CAD build for the part. Positions are in the model's coordinates, mm. Face numbers are marked on the shaded views. A direction names the side the tool comes from. Coordinates: 2 decimals unless noted, no trailing zeros. Write each loop counter-clockwise with the first axis right and the second up, starting at its lowest first coordinate (ties: lowest second). Pieces come first, ordered by that corner, then holes. Notation, with made-up numbers: (86.25, -30.75) -> (140.25, -30.75) arc R9 cw to (140.25, -15.75) -> close; hole circle Ø10 at (25.25, -24). An arc over 180 degrees is marked (long way). Answer as CSV lines item,"result".
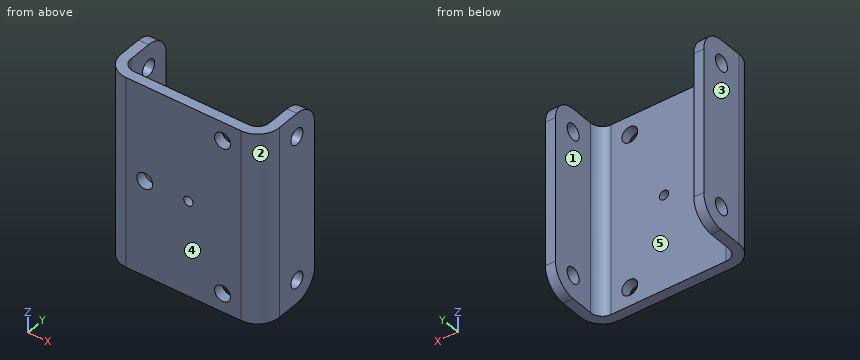
```python
from build123d import *

# Parameters (mm, degrees)
F1_DEPTH = 32.5777606
F2_R     = 3.69316
F3_R     = 1.98374
F4_R     = 1.35255
F5_DEPTH = 26.9875
F6_R     = 3.96875
F7_R     = 0.79375
F7_R_2   = 1.35255
F8_DEPTH = 1.70942


with BuildPart() as f1:
    # F0 (on Top) → F1 (new body)
    with BuildSketch(Plane.XY):
        Polygon((0, 9.92124), (0, 0), (-23.56866, 0), (-23.56866, 9.92124), (-25.27808, 9.92124), (-25.27808, -1.70942), (1.70942, -1.70942), (1.70942, 9.92124), align=None)
    extrude(amount=F1_DEPTH)

    # F2
    f2_edges = [f1.edges().sort_by_distance(p)[0] for p in [
        (1.70942, -1.70942, 16.28888),
        (-25.27808, -1.70942, 16.28888),
    ]]
    fillet(f2_edges, radius=F2_R)

    # F3
    f3_edges = [f1.edges().sort_by_distance(p)[0] for p in [
        (0, 0, 16.28888),
        (-23.56866, 0, 16.28888),
    ]]
    fillet(f3_edges, radius=F3_R)

    # F4 (on face) → F5 (cut, through all)
    with BuildSketch(Plane.YZ.offset(1.70942)):
        with Locations((5.95249, 3.96875)):
            Circle(F4_R)
        with Locations((5.95249, 28.6090106)):
            Circle(F4_R)
    extrude(amount=-F5_DEPTH, mode=Mode.SUBTRACT)

    # F6
    f6_edges = [f1.edges().sort_by_distance(p)[0] for p in [
        (0.85471, 9.92124, 32.577761),
        (-24.42337, 9.92124, 32.577761),
        (0.85471, 9.92124, 0),
        (-24.42337, 9.92124, 0),
    ]]
    fillet(f6_edges, radius=F6_R)

    # F7 (on face) → F8 (cut, through all)
    with BuildSketch(Plane.XZ.offset(1.70942)):
        with Locations((-10.99058, 16.2888803)):
            Circle(F7_R)
        with Locations((-18.40992, 16.2888803)):
            Circle(F7_R_2)
        with Locations((-5.15874, 29.4027606)):
            Circle(F7_R_2)
        with Locations((-5.15874, 3.175)):
            Circle(F7_R_2)
    extrude(amount=-F8_DEPTH, mode=Mode.SUBTRACT)


solid = f1.part
```
Item 1: 3-axis set-ups, long thin cutter, end or side, ignore diameter. For the marked faces 1 and 2: which of +Z, -Z, +X, -X, +Y, -Y reach the whole face in a straight line?
Answer below:
face 1,"+Z, -Z, +Y"
face 2,"+Z, -Z, +X, -Y"
Item 2: Saw through at B-B on x = -4.75. Give the cut face in (y, z).
Answer below:
outline,"(-1.71, 0) -> (0, 0) -> (0, 1.89) -> (-1.71, 1.89) -> close; (-1.71, 4.46) -> (0, 4.46) -> (0, 28.11) -> (-1.71, 28.11) -> close; (-1.71, 30.69) -> (0, 30.69) -> (0, 32.58) -> (-1.71, 32.58) -> close"
Item 3: Saw through at C-C on y = 8.75. Give the cut face in (x, z), and give its area (3 significant figures).
Answer below:
outline,"(-25.28, 1.15) -> (-23.57, 1.15) -> (-23.57, 31.42) -> (-25.28, 31.42) -> close; (0, 1.15) -> (1.71, 1.15) -> (1.71, 31.42) -> (0, 31.42) -> close"
area,"103 mm2"
Item 4: Flat gauge pins, fed straight in: pin 1 (10 mm diameter, centred on x = -13.5, z = 24, fed in from +Y); pin 2 (1 mm diameter, centred on x = -10.99, z = 16.29, fed in from -Y). Where does each tip first touch, or does it go through?
Answer below:
pin 1,"stops at y = 0"
pin 2,"passes through"
Item 5: Wall check: line 1 (X direction, y = 9.5, z = 27); line 2 (Y direction, x = -13, z = 18); line 3 (Z direction, x = -18.5, y = -0.5). Give the ranges that are in metal, low to high. Write a range as from..to.
Answer below:
line 1,"x = -25.28..-23.57, 0..1.71"
line 2,"y = -1.71..0"
line 3,"z = 0..14.94, 17.64..32.58"
Item 6: Saw through at D-D on z = 19.5. Give the cut face in (x, y).
Answer below:
outline,"(-25.28, 1.98) arc R3.69 ccw to (-21.58, -1.71) -> (-1.98, -1.71) arc R3.69 ccw to (1.71, 1.98) -> (1.71, 9.92) -> (0, 9.92) -> (0, 1.98) arc R1.98 cw to (-1.98, 0) -> (-21.58, 0) arc R1.98 cw to (-23.57, 1.98) -> (-23.57, 9.92) -> (-25.28, 9.92) -> close"
Item 7: Saw through at A-A on y = 5. Give the cut face in (x, z), and give its area (3 significant figures).
Answer below:
outline,"(-25.28, 0) -> (-23.57, 0) -> (-23.57, 3.01) -> (-25.28, 3.01) -> close; (-25.28, 4.93) -> (-23.57, 4.93) -> (-23.57, 27.65) -> (-25.28, 27.65) -> close; (-25.28, 29.57) -> (-23.57, 29.57) -> (-23.57, 32.58) -> (-25.28, 32.58) -> close; (0, 0) -> (1.71, 0) -> (1.71, 3.01) -> (0, 3.01) -> close; (0, 4.93) -> (1.71, 4.93) -> (1.71, 27.65) -> (0, 27.65) -> close; (0, 29.57) -> (1.71, 29.57) -> (1.71, 32.58) -> (0, 32.58) -> close"
area,"98.2 mm2"
Item 8: Two-plate mould, pull along X, no slides. Class the marked faces 3, 4 and 5: pulls with the +X half, pulls with the -X half, needs draft (parallel to the pull), parting line crosses it, or undercut.
Answer below:
face 3,"pulls with the -X half"
face 4,"needs draft"
face 5,"undercut"
